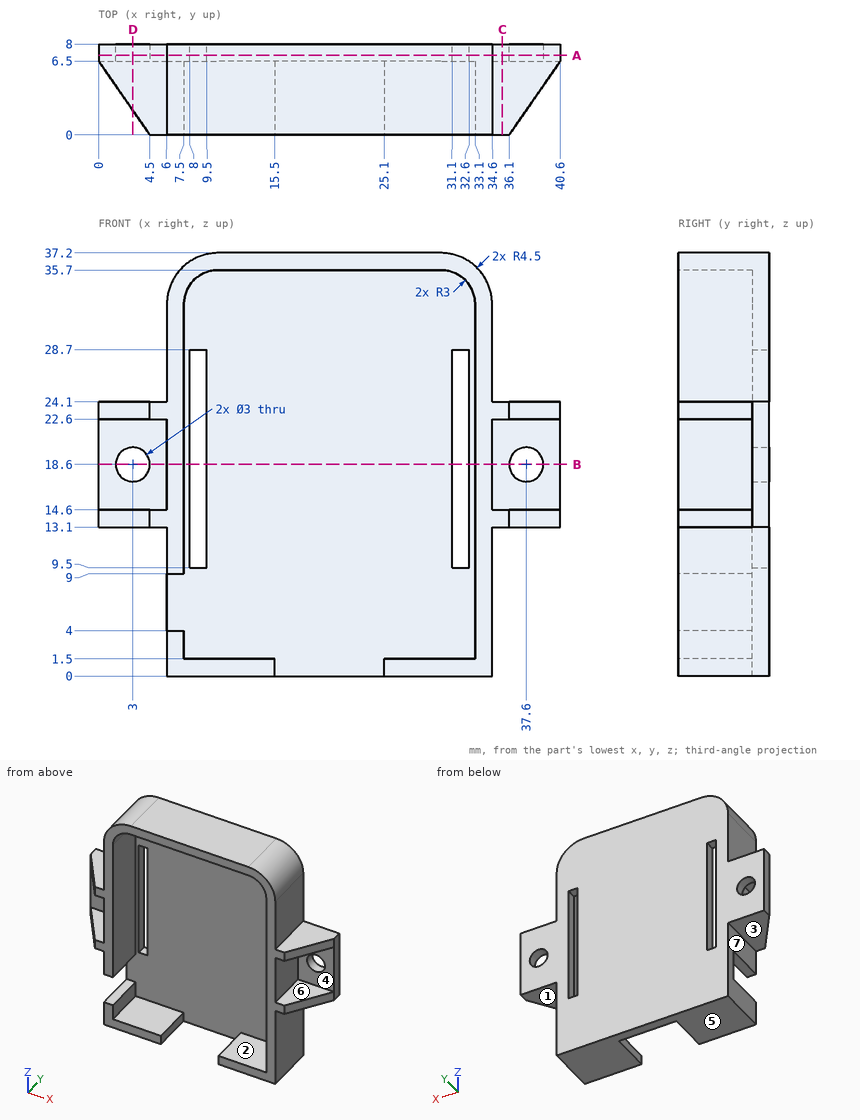
Source: three-view drawing plus pictorial views. Frame: mm from the lowest corner of the part. A direction names the side the tool comes from. Round coordinates to 2 decimals unless told otherwise and drop trailing zeros. Loops run counter-clockwise (first coordinate to the right, second up) from the corner with the lowest first, then second, coordinate; pieces in that order, holes last.
Q1. Access query for the marked faces 1, 2, 3 and 4. Directions: +Z, -Z, +X, -X, +Y, -Y. A direction counts if a zero-diameter tool reaches every point of the face in a straight line with its end or side. Return the directions, or none.
Q2. Section D-D on x = 3. Return loops of the section in (y, z).
Q3. Pull-direction query (Z, two-part tool) for the marked faces 5, 6 and 7; classes: released by +Z, released by -Z, zero draft, split by the parting line, or undercut.
Q4. Section A-A on y = 7. Return loops of the section in (x, z), plus the area to 3 significant figures.
Q5. Section B-B on z = 18.6. Return loops of the section in (x, y), plus the area to 3 significant figures.
Q6. Pin query (flat end, axial travel): P1, Ø1, axis at x = 31.5, y = 1, coming from the +Z side; P2, Ø2, axis at y = 1.5, z = 17, coming from the +X side; P3, Ø3, axis at y = 4.5, z = 16.5, coming from the -X side. Return the tip coordinate at first contact, or that it passes through.
Q7. Material intervals for L1, parallel to X at y = 7.25, z = 23.5; L2, parallel to Z at x = 37.6, y = 7.75; L3, parallel to X at y = 1.5, z = 12.5, sorted ascending.
Q8. Section C-C on x = 35.5. Return loops of the section in (y, z), plus the area to 3 significant figures.
Evaluation:
1. face 1: -Z, +X, +Y, -Y
1. face 2: -Y
1. face 3: -Z, -X, +Y, -Y
1. face 4: +X, -Y
2. outline: (2.17, 13.1) - (8, 13.1) - (8, 17.1) - (6.5, 17.1) - (6.5, 14.6) - (2.17, 14.6) - close; (2.17, 22.6) - (6.5, 22.6) - (6.5, 20.1) - (8, 20.1) - (8, 24.1) - (2.17, 24.1) - close
3. face 5: released by -Z
3. face 6: undercut
3. face 7: zero draft
4. outline: (0, 13.1) - (6, 13.1) - (6, 0) - (34.6, 0) - (34.6, 13.1) - (40.6, 13.1) - (40.6, 24.1) - (34.6, 24.1) - (34.6, 32.7) arc R4.5 ccw to (30.1, 37.2) - (10.5, 37.2) arc R4.5 ccw to (6, 32.7) - (6, 24.1) - (0, 24.1) - close; hole circle Ø3 at (3, 18.6); hole (8, 9.5) - (9.5, 9.5) - (9.5, 28.7) - (8, 28.7) - close; hole (31.1, 9.5) - (32.6, 9.5) - (32.6, 28.7) - (31.1, 28.7) - close; hole circle Ø3 at (37.6, 18.6)
4. area: 1,120 mm2
5. outline: (0, 6.5) - (1.5, 6.5) - (1.5, 8) - (0, 8) - close; (4.5, 6.5) - (6, 6.5) - (6, 0) - (7.5, 0) - (7.5, 6.5) - (8, 6.5) - (8, 8) - (4.5, 8) - close; (9.5, 6.5) - (31.1, 6.5) - (31.1, 8) - (9.5, 8) - close; (32.6, 6.5) - (33.1, 6.5) - (33.1, 0) - (34.6, 0) - (34.6, 6.5) - (36.1, 6.5) - (36.1, 8) - (32.6, 8) - close; (39.1, 6.5) - (40.6, 6.5) - (40.6, 8) - (39.1, 8) - close
5. area: 66.9 mm2
6. P1: stops at z = 37.11
6. P2: stops at x = 34.6
6. P3: stops at x = 6
7. L1: x = 0 to 8, 9.5 to 31.1, 32.6 to 40.6
7. L2: z = 13.1 to 17.1, 20.1 to 24.1
7. L3: x = 6 to 7.5, 33.1 to 34.6
8. outline: (0, 13.1) - (8, 13.1) - (8, 24.1) - (0, 24.1) - (0, 22.6) - (6.5, 22.6) - (6.5, 14.6) - (0, 14.6) - close
8. area: 36.0 mm2
